from build123d import *

# Parameters (mm, degrees)
SKETCH1_R                = 15
SKETCH1_R_2              = 7.5
BOSS_EXTRUDE1_DEPTH      = 152.5
BOSS_EXTRUDE1_DEPTH_BACK = 152.5
SKETCH2_R                = 3.1
CUT_EXTRUDE1_DEPTH       = 16
SKETCH3_R                = 3.1
CUT_EXTRUDE2_DEPTH       = 16.000000102


with BuildPart() as part:
    # Sketch1 → Boss-Extrude1 (new body, two sides)
    with BuildSketch(Plane.XY) as boss_extrude1_sk:
        Circle(SKETCH1_R)
        Circle(SKETCH1_R_2, mode=Mode.SUBTRACT)
    extrude(amount=BOSS_EXTRUDE1_DEPTH)
    extrude(boss_extrude1_sk.sketch, amount=-BOSS_EXTRUDE1_DEPTH_BACK)

    # Sketch2 → Cut-Extrude1 (cut, through all)
    with BuildSketch(Plane(origin=(0, 0, 0), x_dir=(1, 0, 0), z_dir=(0, 1, 0))):
        with Locations((0, -112.5)):
            Circle(SKETCH2_R)
    extrude(amount=CUT_EXTRUDE1_DEPTH, mode=Mode.SUBTRACT)

    # Sketch3 → Cut-Extrude2 (cut, through all)
    with BuildSketch(Plane(origin=(0, 0, 0), x_dir=(1, 0, 0), z_dir=(0, 1, 0))):
        with Locations((0, 137.5)):
            Circle(SKETCH3_R)
    extrude(amount=CUT_EXTRUDE2_DEPTH, mode=Mode.SUBTRACT)


solid = part.part
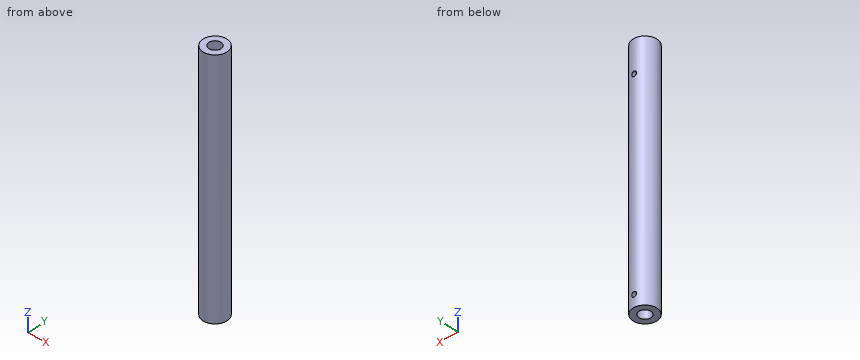
Check sheet for the modelled part. Datum: model origin and axes. Units: mm. Coordinates: 2 decimals unless noted, no trailing zeros. Loops run counter-clockwise (first coordinate to the right, second up) from the corner with the lowest first, then second, coordinate; pieces in that order, holes last. Notation, with made-up numbers: (-6.5, -25.75) -> (0.5, -25.75) arc R16 ccw to (0.5, -13.75) -> close; hole circle Ø9 at (52.25, 68). An arc over 180 degrees is marked (long way). Answer in a Markdown table with one row per item.
1. Sectioned sample at D-D, the plane x = -11.5. Record the boundary of the cut face in (y, z), then the cut area to 3 significant figures.
Check values:
| item | result |
|---|---|
| outline | (-9.63, -152.5) -> (9.63, -152.5) -> (9.63, 152.5) -> (-9.63, 152.5) -> close |
| area | 5,870 mm2 |
2. Material ranges on line 1 along Z through (x, y) = (0, 9); line 2 along Z through (x, y) = (2.5, 13.5); line 3 along X through (y, z) = (10, -137.5), recorded low to high. Write a range as [from, to].
Check values:
| item | result |
|---|---|
| line 1 | z = [-152.5, -140.6], [-134.4, 109.4], [115.6, 152.5] |
| line 2 | z = [-152.5, -139.33], [-135.67, 110.67], [114.33, 152.5] |
| line 3 | x = [-11.18, -3.1], [3.1, 11.18] |
3. Go/stop test with flat-tipped pins: pin 1 (8 mm diameter, centred on x = 4.5, y = 3, fed in from -Z); pin 2 (1 mm diameter, centred on x = 9.5, z = -116, fed in from +Y); pin 3 (5 mm diameter, centred on y = 8.5, z = -64.5, fed in from -X); pin 4 (12 mm diameter, centred on x = -11, z = 57, fed in from -Y). Record where each tip stops, or that it passes through.
Check values:
| item | result |
|---|---|
| pin 1 | stops at z = -152.5 |
| pin 2 | stops at y = 12 |
| pin 3 | stops at x = -13.75 |
| pin 4 | stops at y = -14.14 |
4. Sectioned sample at B-B, the plane y = 0. Record the boundary of the cut face in (x, z), then the cut area to 4 significant figures.
Check values:
| item | result |
|---|---|
| outline | (-15, -152.5) -> (-7.5, -152.5) -> (-7.5, 152.5) -> (-15, 152.5) -> close; (7.5, -152.5) -> (15, -152.5) -> (15, 152.5) -> (7.5, 152.5) -> close |
| area | 4,575 mm2 |
5. Sectioned sample at C-C, the plane z = -85.5. Record the boundary of the cut face in (x, y), then the cut area to 3 significant figures.
Check values:
| item | result |
|---|---|
| outline | circle Ø30 at (0, 0); hole circle Ø15 at (0, 0) |
| area | 530 mm2 |
6. Sectioned sample at A-A, the plane x = 0. Record the boundary of the cut face in (y, z).
Check values:
| item | result |
|---|---|
| outline | (-15, -152.5) -> (-7.5, -152.5) -> (-7.5, 152.5) -> (-15, 152.5) -> close; (7.5, -152.5) -> (15, -152.5) -> (15, -140.6) -> (7.5, -140.6) -> close; (7.5, -134.4) -> (15, -134.4) -> (15, 109.4) -> (7.5, 109.4) -> close; (7.5, 115.6) -> (15, 115.6) -> (15, 152.5) -> (7.5, 152.5) -> close |
